from build123d import *

# Parameters (mm, degrees)
SKETCH1_W           = 27.6
SKETCH1_H           = 27.6
BOSS_EXTRUDE1_DEPTH = 9.8
CUT_EXTRUDE1_DEPTH  = 44.676996234
SKETCH3_W           = 15.2
SKETCH3_H           = 24.2
CUT_EXTRUDE2_DEPTH  = 24.2
CUT_EXTRUDE3_DEPTH  = 44.676996234
FILLET110_R         = 2
CUT_EXTRUDE4_DEPTH  = 38.992630864
CUT_EXTRUDE5_DEPTH  = 38.992630864
SKETCH7_W           = 5.8
SKETCH7_H           = 3
BOSS_EXTRUDE2_DEPTH = 2
SKETCH8_W           = 5.8
SKETCH8_H           = 3
BOSS_EXTRUDE3_DEPTH = 2
CUT_EXTRUDE6_DEPTH  = 42.046437117
TAP101_D            = 4.134


with BuildPart() as part:
    # Sketch1 → Boss-Extrude1 (new, symmetric)
    with BuildSketch(Plane(origin=(0, 0, 0), x_dir=(0, 0, -1), z_dir=(1, 0, 0))):
        with Locations((-13.8, 13.8)):
            Rectangle(SKETCH1_W, SKETCH1_H)
    extrude(amount=BOSS_EXTRUDE1_DEPTH, both=True)

    # Sketch2 → Cut-Extrude1 (cut, through all)
    with BuildSketch(Plane.ZY.offset(9.8)):
        Polygon((27.6, 27.6), (5.4, 27.6), (27.6, 5.4), align=None)
    extrude(amount=-CUT_EXTRUDE1_DEPTH, mode=Mode.SUBTRACT)

    # Sketch3 → Cut-Extrude2 (cut)
    with BuildSketch(Plane(origin=(0, 27.6, 0), x_dir=(1, 0, 0), z_dir=(0, 1, 0))):
        with Locations((0, -15.5)):
            Rectangle(SKETCH3_W, SKETCH3_H)
    extrude(amount=-CUT_EXTRUDE2_DEPTH, mode=Mode.SUBTRACT)

    # Sketch4 → Cut-Extrude3 (cut, through all)
    with BuildSketch(Plane.ZY.offset(9.8)):
        Polygon((5.4, 27.6), (5.4, 21.2), (21.2, 5.4), (27.6, 5.4), align=None)
    extrude(amount=-CUT_EXTRUDE3_DEPTH, mode=Mode.SUBTRACT)

    # Fillet110
    fillet110_edges = [part.edges().sort_by_distance(p)[0] for p in [
        (8.7, 5.4, 27.6),
        (-8.7, 5.4, 27.6),
        (8.7, 27.6, 5.4),
        (-8.7, 27.6, 5.4),
    ]]
    fillet(fillet110_edges, radius=FILLET110_R)

    # Sketch5 → Cut-Extrude4 (cut, through all)
    with BuildSketch(Plane.XY.offset(3.4)):
        with BuildLine():
            Line((-3.4, 14.7), (-3.4, 18.3))
            ThreePointArc((-3.4, 18.3), (0, 21.7), (3.4, 18.3))
            Line((3.4, 18.3), (3.4, 14.7))
            ThreePointArc((3.4, 14.7), (0, 11.3), (-3.4, 14.7))
        make_face()
    extrude(amount=-CUT_EXTRUDE4_DEPTH, mode=Mode.SUBTRACT)

    # Sketch6 → Cut-Extrude5 (cut, through all)
    with BuildSketch(Plane(origin=(0, 3.4, 0), x_dir=(1, 0, 0), z_dir=(0, 1, 0))):
        with BuildLine():
            Line((3.4, -14.7), (3.4, -18.3))
            ThreePointArc((3.4, -18.3), (0, -21.7), (-3.4, -18.3))
            Line((-3.4, -18.3), (-3.4, -14.7))
            ThreePointArc((-3.4, -14.7), (0, -11.3), (3.4, -14.7))
        make_face()
    extrude(amount=-CUT_EXTRUDE5_DEPTH, mode=Mode.SUBTRACT)

    # Sketch7 → Boss-Extrude2 (add)
    with BuildSketch(Plane(origin=(0, 0, 0), x_dir=(-1, 0, 0), z_dir=(0, 0, -1))):
        with Locations((0, 24.6)):
            Rectangle(SKETCH7_W, SKETCH7_H)
        with Locations((0, 3)):
            Rectangle(SKETCH7_W, SKETCH7_H)
    extrude(amount=BOSS_EXTRUDE2_DEPTH)

    # Sketch8 → Boss-Extrude3 (add)
    with BuildSketch(Plane.XZ):
        with Locations((0, 24.6)):
            Rectangle(SKETCH8_W, SKETCH8_H)
        with Locations((0, 3)):
            Rectangle(SKETCH8_W, SKETCH8_H)
    extrude(amount=BOSS_EXTRUDE3_DEPTH)

    # Sketch9 → Cut-Extrude6 (cut, through all)
    with BuildSketch(Plane(origin=(2.9, 0, 0), x_dir=(0, 0, -1), z_dir=(1, 0, 0))):
        Polygon((0, 26.1), (2, 23.6), (2, 26.1), align=None)
        Polygon((0, 4.5), (2, 4.5), (2, 2), align=None)
        Polygon((-26.1, 0), (-26.1, -2), (-23.6, -2), align=None)
        Polygon((-4.5, 0), (-4.5, -2), (-2, -2), align=None)
    extrude(amount=-CUT_EXTRUDE6_DEPTH, mode=Mode.SUBTRACT)

    # Tap101 (through all)
    with Locations(Plane.ZY.offset(9.8)):
        with Locations((8, 8)):
            Hole(TAP101_D / 2)


solid = part.part
Geometry: final body of the model. Coordinates: model frame, mm. A direction names the side the tool comes from. Coordinates: 2 decimals unless noted, no trailing zeros. Loops run counter-clockwise (first coordinate to the right, second up) from the corner with the lowest first, then second, coordinate; pieces in that order, holes last. Notation, with made-up numbers: M 25.5,72.5 L 32.5,72.5 A12 ccw 32.5,87.5 Z; hole C 84,-38.5 d8. An arc over 180 degrees is marked long. One line per item, written item: value. Start each with the question number.
1) Material intervals for L1, parallel to X at y = 12.5, z = 4.5; L2, parallel to Z at x = -8, y = 2.75; L3, parallel to X at y = 2.5, z = 18.25, sorted ascending. Write a range as from..to.
2) Reachability of faces 4 (the flat face through (-3.4, 16, 2)), 5 (the flat face through (-7.6, 10, 10)), 6 (the flat face through (0, 23.1, -1)), 7 (the cylindrical face through (0.1, 1.7, 21.7)) from +Z, -Z, +X, -X, +Y, -Y: full face, straight path, thin tool, end or side. Return the list, or none.
3) Cut plane D-D (z = 13.5). Return loops of the section in (x, y), then the cut area to 3 significant figures.
4) Draft query along X for faces 1 (the flat face through (3.4, 2, 16)), 2 (the flat face through (2.9, -1, 3)), 3 (the flat face through (0, -1, 23.1)). Return one class per face: released by +X, released by -X, zero draft, split by the parting line, or undercut.
5) Cut plane C-C (x = 0). Count the separate pieces of the cut face and the enclosed holes in it, then the cut area to 3 significant figures.
6) Pin query (flat end, axial travel): P1, Ø1.5, axis at x = 6, z = 4, coming from the -Y side; P2, Ø1.6, axis at y = 24.5, z = -1.5, coming from the +X side; P3, Ø4, axis at x = -4.5, y = 22.5, coming from the +Z side; P4, Ø3.5, axis at y = 8, z = 8, coming from the -X side. Return the tip coordinate at first contact, or that it passes through.
7) Cut plane A-A (z = 8). Return loops of the section in (x, y).
Evaluation:
1. L1: -9.8..-7.6, 7.6..9.8
1. L2: 0..27.6
1. L3: -9.8..-3.4, 3.4..9.8
2. face 4: +Z, -Z
2. face 5: +Z, +Y
2. face 6: -Z, +X, -X
2. face 7: +Y, -Y
3. outline: M -9.8,0 L -3.18,0 L -3.18,3.4 L -7.6,3.4 L -7.6,13.1 L -9.8,13.1 Z; M 3.18,0 L 9.8,0 L 9.8,13.1 L 7.6,13.1 L 7.6,3.4 L 3.18,3.4 Z
3. area: 87.7 mm^2
4. face 1: undercut
4. face 2: released by +X
4. face 3: zero draft
5. separate pieces: 3
5. enclosed holes: 0
5. area: 119 mm^2
6. P1: y = 0
6. P2: x = 2.9
6. P3: z = 3.4
6. P4: through
7. outline: M -9.8,0 L 9.8,0 L 9.8,5.93 L 7.6,5.93 L 7.6,3.4 L -7.6,3.4 L -7.6,5.93 L -9.8,5.93 Z; M -9.8,10.07 L -7.6,10.07 L -7.6,18.6 L -9.8,18.6 Z; M 7.6,10.07 L 9.8,10.07 L 9.8,18.6 L 7.6,18.6 Z
